```python
from build123d import *

# Parameters (mm, degrees)
SKETCH_1_R      = 13.585
EXTRUDE_1_DEPTH = 62


with BuildPart() as part:
    # 草图1 → 凸台-拉伸1 (new body)
    with BuildSketch(Plane(origin=(0, 0, 0), x_dir=(1, 0, 0), z_dir=(0, 1, 0))):
        with Locations(Location((0, 0, 0), (0, 0, 270))):
            Circle(SKETCH_1_R)
    extrude(amount=EXTRUDE_1_DEPTH)

    # 草图2 → 旋转1 (revolve)
    with BuildSketch(Plane.XY, mode=Mode.PRIVATE) as revolve_1_sk:
        Polygon((2.339013215, -6), (2.739013215, -6), (3.339013215, -4), (2.739013215, -4), (3.339013215, -2), (2.739013215, -2), (3.339013215, 0), (2.339013215, 0), align=None)
    revolve(revolve_1_sk.sketch.rotate(Axis((0, 0, 0), (0, -1, 0)), 90), axis=Axis((0, 0, 0), (0, -1, 0)))


solid = part.part
```
Work out the finished part from the listing and answer in its coordinate system (mm). A direction names the side the tool comes from. Give positions to 0.01 mm unless a question says otherwise; leave off trailing zeros. Order: outer loops, then holes, each group sorted by start corner. A loop starts at its lowest first (then second) coordinate and runs counter-clockwise, first axis right, second up. Notation, with made-up numbers: (54, 80) - (110, 80) arc R8 ccw to (110, 88) - close; hole circle Ø5 at (-24, -22.75). An arc over 180 degrees is marked (long way). One line per item, written item: value. Start each with the question number.
1. Consider line 1 (Y direction, x = 4.5, z = 12.75); line 2 (X direction, y = -1.35, z = 0); line 3 (X direction, y = -4.6, z = 0). Determine where each line is inside the solid, lowest interval first.
2. Each of these flat-tipped pins is pushed along its axis until it touches: pin 1 Ø1 at (x, y) = (-2, 53) entering from +Z; pin 2 Ø1.5 at (x, y) = (10.5, 24) entering from -Z; pin 3 Ø1 at (x, z) = (7.5, -3.5) entering from -Y. Where does it stop, or does it pass through?
3. Section B-B, the plane z = 0 is taken. Write down the section's boundary in (x, y) (3 decimals), then the cut area to 3 significant figures.
4. Which of the six approach directions +Z, -Z, +X, -X, +Y, -Y give full straight-line access (tool end or side, diameter ignored) to faces 5 (the face through (2.283, -3.042, -0.507)), 6 (the face through (0, 62, 0))?
5. Section C-C, the plane y = 8.5 is taken. Write down the section's boundary in (x, z) (3 decimals), then the cut area to 3 significant figures.
6. Section D-D, the plane z = -8.75 is taken. Write down the section's boundary in (x, y).
7. For a pull along Y with two mould halves and no side action, classify faces 1 (the face through (0, 0, 0)), 2 (the face through (13.47, 30.57, -1.77)), 3 (the face through (-3, -2, 0)), 4 (the face through (-3, -4, 0)) as released by +Y, released by -Y, zero draft, split by the parting line, or undercut.
8. Section A-A, the plane x = 0 is taken. Write down the section's boundary in (y, z) (3 decimals), then the cut area to 3 significant figures.
Filled sheet:
1. line 1: 0 to 62
1. line 2: -2.93 to -2.34, 2.34 to 2.93
1. line 3: -3.16 to -2.34, 2.34 to 3.16
2. pin 1: z = 13.5
2. pin 2: z = -9.46
2. pin 3: y = 0
3. outline: (-13.585, 0) - (-3.339, 0) - (-2.739, -2) - (-3.339, -2) - (-2.739, -4) - (-3.339, -4) - (-2.739, -6) - (-2.339, -6) - (-2.339, 0) - (2.339, 0) - (2.339, -6) - (2.739, -6) - (3.339, -4) - (2.739, -4) - (3.339, -2) - (2.739, -2) - (3.339, 0) - (13.585, 0) - (13.585, 62) - (-13.585, 62) - close
3. area: 1,690 mm²
4. face 5: -Y
4. face 6: +Z, -Z, +X, -X, +Y
5. outline: circle Ø27.17 at (0, 0)
5. area: 580 mm²
6. outline: (-10.39, 0) - (10.39, 0) - (10.39, 62) - (-10.39, 62) - close
7. face 1: released by -Y
7. face 2: zero draft
7. face 3: undercut
7. face 4: undercut
8. outline: (-6, -2.739) - (-4, -3.339) - (-4, -2.739) - (-2, -3.339) - (-2, -2.739) - (0, -3.339) - (0, -13.585) - (62, -13.585) - (62, 13.585) - (0, 13.585) - (0, 3.339) - (-2, 2.739) - (-2, 3.339) - (-4, 2.739) - (-4, 3.339) - (-6, 2.739) - (-6, 2.339) - (0, 2.339) - (0, -2.339) - (-6, -2.339) - close
8. area: 1,690 mm²
